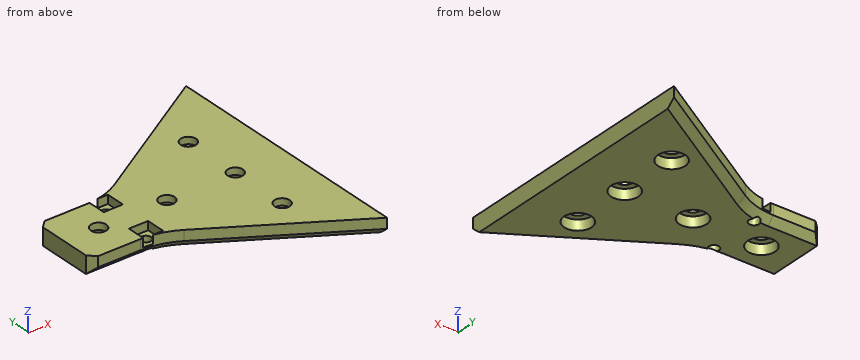
Autodesk Inventor part; units mm, degrees
ref_plane "YZ Plane" through (0, 0, 0) normal (1, 0, 0) x (0, 1, 0)
ref_plane "XZ Plane" through (0, 0, 0) normal (0, 1, 0) x (-1, 0, 0)
ref_plane "XY Plane" through (0, 0, 0) normal (0, 0, 1) x (1, 0, 0)
sketch "Sketch1" plane through (0, 0, 0) normal (0, 0, 1) x (1, 0, 0)
  line L0 (0, 0) -> (-50, 0) construction
  line L1 (-50, 0) -> (-50, 10)
  line L2 (-50, 0) -> (-50, -10)
  line L3 (-50, -10) -> (-30, -10)
  line L4 (-30, -10) -> (15, -37.5)
  line L5 (-50, 10) -> (-30, 10)
  line L6 (-30, 10) -> (15, 37.5)
  line L7 (15, 37.5) -> (15, -37.5)
  line L8 (0, 0) -> (15, 0) construction
  line L9 (0, 17.5) -> (0, -17.5) construction
  point P0 (-40, 0)
  point P1 (-20, 0)
  dimension "d0" = 20
  dimension "d1" = 65
  dimension "d2" = 50
  dimension "d4" = 20
  dimension "d5" = 75
  dimension "d6" = 35
  dimension "d9" = 40
  dimension "d41" = 20
extrude "Extrusion1" add sketch "Sketch1" along normal blind 5
hole "Hole1" at (0, 17.5, 0) at (0, -17.5, 0) at (-40, 0, 0) at (0, 0, 0) at (-20, 0, 0) direction (0, 0, 1) diameter 4.5 end through all counterbore diameter 8 counterbore depth 3
fillet "Fillet1" radius 20 2 edges at (-30, 10, 2.5) (-30, -10, 2.5)
chamfer "Chamfer1" distance 2 angle 45 2 edges at (-50, 10, 2.5) (-50, -10, 2.5)
sketch "Sketch2" plane through (0, 0, 0) normal (0, 0, -1) x (-1, 0, 0)
  line L0 (50, -8) -> (48, -10)
  line L1 (50, 8) -> (50, -8)
  line L2 (48, 10) -> (50, 8)
  line L3 (35.6273, 10) -> (48, 10)
  arc A0 (25.1983, 12.9344) -> (35.6273, 10) centre (35.6273, 30) ccw
  line L4 (-15, 37.5) -> (25.1983, 12.9344)
  line L5 (-15, -37.5) -> (-15, 37.5)
  line L6 (25.1983, -12.9344) -> (-15, -37.5)
  arc A1 (35.6273, -10) -> (25.1983, -12.9344) centre (35.6273, -30) ccw
  line L7 (48, -10) -> (35.6273, -10)
  circle A2 centre (0, 0) radius 4
  circle A3 centre (40, 0) radius 4
  circle A4 centre (0, -17.5) radius 4
  circle A5 centre (0, 17.5) radius 4
  line L8 (32, 7.5) -> (32, -7.5) construction
  line L9 (50, 0) -> (32, 0) construction
  circle A6 centre (32, 7.5) radius 1.5
  circle A7 centre (32, -7.5) radius 1.5
  line L10 (29, 4) -> (32, 4)
  line L11 (32, 4) -> (32, -4)
  line L12 (32, -4) -> (29, -4)
  line L13 (29, -4) -> (29, 4)
  line L14 (50, 4) -> (47, 4)
  line L15 (47, 4) -> (47, -4)
  line L16 (47, -4) -> (50, -4)
  line L17 (50, -4) -> (50, 4)
  line L18 (50, 8) -> (50, -8)
  point P0 (32, 0)
  point P1 (47, 0)
  dimension "d24" = 18
  dimension "d25" = 15
  dimension "d26" = 3
  dimension "d27" = 3
  dimension "d30" = 3
  dimension "d31" = 3
  dimension "d32" = 8
  dimension "d33" = 8
  dimension "d34" = 3
extrude "Extrusion2" cut sketch "Sketch2" against normal through all contours A6 | A7
chamfer "Chamfer2" distance 2 angle 45 6 edges at (-41.8137, 10, 0) (-30.2103, 10.7476, 0) (-5.0992, 25.2172, 0) (-30.2103, -10.7476, 0) (-5.0992, -25.2172, 0) (-41.8137, -10, 0)
sketch "Sketch3" plane through (0, 0, 5) normal (0, 0, 1) x (1, 0, 0)
  circle A0 centre (-32, 7.5) radius 1.5
  circle A1 centre (-32, -7.5) radius 1.5
  line L0 (-29.2, 4.7) -> (-34.8, 4.7)
  line L1 (-34.8, 4.7) -> (-34.8, 10.3)
  line L2 (-34.8, 10.3) -> (-29.2, 10.3)
  line L3 (-29.2, 10.3) -> (-29.2, 4.7)
  line L4 (-29.2, 4.7) -> (-34.8, 10.3) construction
  line L5 (-34.8, 4.7) -> (-29.2, 10.3) construction
  line L6 (-29.2, -10.3) -> (-34.8, -10.3)
  line L7 (-34.8, -10.3) -> (-34.8, -4.7)
  line L8 (-34.8, -4.7) -> (-29.2, -4.7)
  line L9 (-29.2, -4.7) -> (-29.2, -10.3)
  line L10 (-29.2, -10.3) -> (-34.8, -4.7) construction
  line L11 (-34.8, -10.3) -> (-29.2, -4.7) construction
  point P0 (0, 0)
  dimension "d37" = 5.6
  dimension "d38" = 5.6
extrude "Extrusion4" cut sketch "Sketch3" against normal blind 2.5
equation "\"d27\" = d26"
properties part number "Y Axis Holder_3DPrint"
Input: part model. Units: mm. Frame: model coordinates. Coordinates: 2 decimals unless noted, no trailing zeros. Loops run counter-clockwise (first coordinate to the right, second up) from the corner with the lowest first, then second, coordinate; pieces in that order, holes last. Notation, with made-up numbers: (61.25, 26.5) -> (119.25, 26.5) arc R22 cw to (119.25, 49.5) -> close; hole circle Ø7 at (-33, -38). An arc over 180 degrees is marked (long way). Use a Markdown table: item, result.
1) Material intervals for line 1 along X through (y, z) = (0, 1.1); line 2 along X through (y, z) = (0, 3.7); line 3 along X through (y, z) = (7, 4.7), sorted ascending. Write a range as from..to.
Results found:
| item | result |
|---|---|
| line 1 | x = -50..-44, -36..-24, -16..-4, 4..15 |
| line 2 | x = -50..-42.25, -37.75..-22.25, -17.75..-2.25, 2.25..15 |
| line 3 | x = -50..-34.8, -29.2..15 |
2) Cut plane B-B (z = 3.85). Return the cut outline in (x, y).
Results found:
| item | result |
|---|---|
| outline | (-50, -8) -> (-48, -10) -> (-35.63, -10) arc R20 cw to (-34.8, -10.02) -> (-34.8, -4.7) -> (-29.2, -4.7) -> (-29.2, -10.3) -> (-32.18, -10.3) arc R20 cw to (-25.2, -12.93) -> (15, -37.5) -> (15, 37.5) -> (-25.2, 12.93) arc R20 cw to (-32.18, 10.3) -> (-29.2, 10.3) -> (-29.2, 4.7) -> (-34.8, 4.7) -> (-34.8, 10.02) arc R20 cw to (-35.63, 10) -> (-48, 10) -> (-50, 8) -> close; hole circle Ø4.5 at (-40, 0); hole circle Ø4.5 at (-20, 0); hole circle Ø4.5 at (0, -17.5); hole circle Ø4.5 at (0, 0); hole circle Ø4.5 at (0, 17.5) |
3) Cut plane D-D (x = -14). Return the cut outline in (y, z).
Results found:
| item | result |
|---|---|
| outline | (-19.78, 2) -> (-17.43, 0) -> (17.43, 0) -> (19.78, 2) -> (19.78, 5) -> (-19.78, 5) -> close |
4) Cut plane A-A (y = 0). Return the cut outline in (x, z).
Results found:
| item | result |
|---|---|
| outline | (-50, 0) -> (-44, 0) -> (-44, 3) -> (-42.25, 3) -> (-42.25, 5) -> (-50, 5) -> close; (-37.75, 3) -> (-36, 3) -> (-36, 0) -> (-24, 0) -> (-24, 3) -> (-22.25, 3) -> (-22.25, 5) -> (-37.75, 5) -> close; (-17.75, 3) -> (-16, 3) -> (-16, 0) -> (-4, 0) -> (-4, 3) -> (-2.25, 3) -> (-2.25, 5) -> (-17.75, 5) -> close; (2.25, 3) -> (4, 3) -> (4, 0) -> (15, 0) -> (15, 5) -> (2.25, 5) -> close |
5) Contact query for flat-ended pins moving along their axis: pin 1 (5 mm diameter, centred on x = -40, y = 0, fed in from -Z); pin 2 (3.5 mm diameter, centred on x = -32, y = 7.5, fed in from +Z); pin 3 (2 mm diameter, centred on y = 9.5, z = 1.5, fed in from -X). Output: stop coordinate, or through.
Results found:
| item | result |
|---|---|
| pin 1 | stops at z = 3 |
| pin 2 | stops at z = 2.5 |
| pin 3 | stops at x = -49.5 |
6) Cut plane C-C (y = -17.5). Return the cut outline in (x, z).
Results found:
| item | result |
|---|---|
| outline | (-17.73, 2) -> (-13.89, 0) -> (-4, 0) -> (-4, 3) -> (-2.25, 3) -> (-2.25, 5) -> (-17.73, 5) -> close; (2.25, 3) -> (4, 3) -> (4, 0) -> (15, 0) -> (15, 5) -> (2.25, 5) -> close |
